Input: dimensioned drawing with shaded views. Units: mm. Origin: part minimum x, y, z. Give positions to 0.01 mm unless a question says otherwise; leave off trailing zeros. Write each loop counter-clockwise with the first axis right and the second up, starting at its lowest first coordinate (ties: lowest second). Pieces come first, ordered by that corner, then holes. Notation, with made-up numbers: M 67.25,61.25 L 79.25,61.25 A37 ccw 79.25,97.25 Z; hole C 15.25,-9 d7. An arc over 180 degrees is marked long. Answer as a JSON object with one key per item and string values.
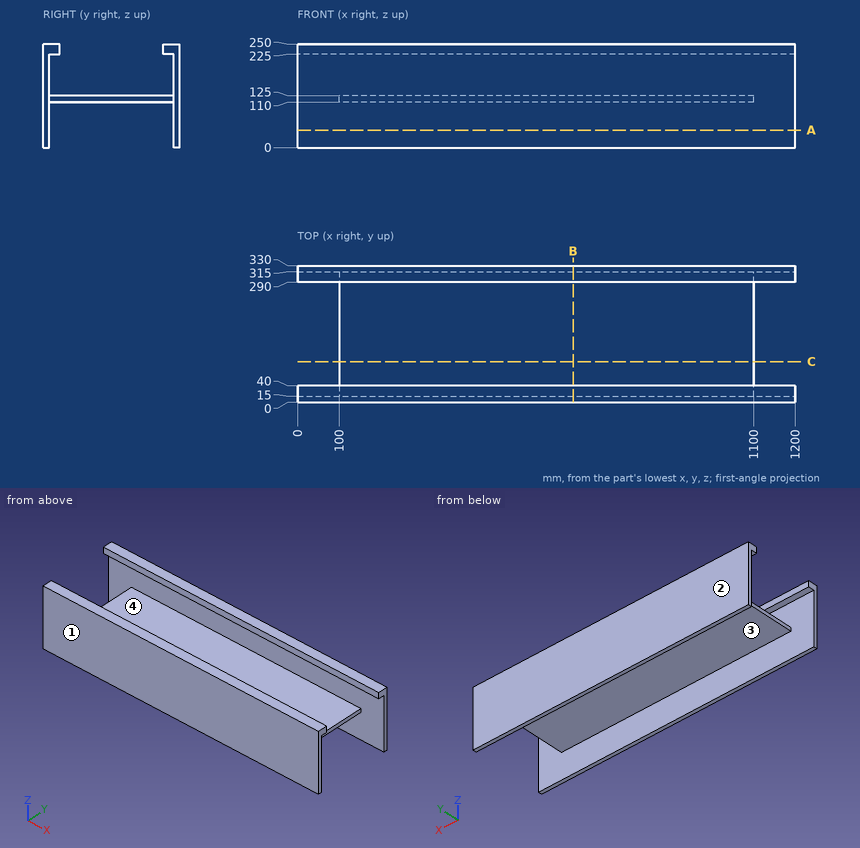
1) Cut plane B-B on x = 664.5. Return loops of the section in (y, z), and give its area (4 significant figures).
Geometry check:
{"outline": "M 0,0 L 15,0 L 15,110 L 315,110 L 315,0 L 330,0 L 330,250 L 290,250 L 290,225 L 315,225 L 315,125 L 15,125 L 15,225 L 40,225 L 40,250 L 0,250 Z", "area": "13,250 mm2"}
2) Line query: line 1 (Z direction, x = 483.5, y = 39); line 2 (Y direction, x = 105, z = 229.5); line 3 (Y direction, x = 449, z = 24). Output: solid intervals per line, ascending. Write a range as from..to.
Geometry check:
{"line 1": "z = 110..125, 225..250", "line 2": "y = 0..40, 290..330", "line 3": "y = 0..15, 315..330"}
3) Cut plane C-C on y = 98.5. Return loops of the section in (x, z).
Geometry check:
{"outline": "M 100,110 L 1100,110 L 1100,125 L 100,125 Z"}
4) Contact query for flat-ended pins moving along their axis: P1, Ø1.5, axis at x = 216, y = 250.5, coming from the -Z side; P2, Ø20, axis at x = 520.5, z = 232.5, coming from the -Y side; P3, Ø7.5, axis at y = 129.5, z = 120.5, coming from the +X side; P4, Ø7.5, axis at y = 144, z = 120.5, coming from the -X side. Output: stop coordinate, or through.
Geometry check:
{"P1": "stops at z = 110", "P2": "stops at y = 0", "P3": "stops at x = 1100", "P4": "stops at x = 100"}
5) Cut plane A-A on z = 42. Return loops of the section in (x, y), and give its area (3 significant figures).
Geometry check:
{"outline": "M 0,0 L 1200,0 L 1200,15 L 0,15 Z; M 0,315 L 1200,315 L 1200,330 L 0,330 Z", "area": "36,000 mm2"}
6) Pull-direction query (Y, two-part tool) for the marked faces 1, 2, 3 and 4; classes: pulls with the +Y half, pulls with the -Y half, needs draft (parallel to the pull), parting line crosses it, or undercut.
Geometry check:
{"face 1": "pulls with the -Y half", "face 2": "pulls with the +Y half", "face 3": "undercut", "face 4": "undercut"}
